from build123d import *

# Parameters (mm, degrees)
SKETCH_1_R      = 1
EXTRUDE_1_DEPTH = 1.5
SKETCH_2_W      = 30
SKETCH_2_H      = 14
EXTRUDE_2_DEPTH = 7.5
SKETCH_3_W      = 8
SKETCH_3_H      = 12
EXTRUDE_3_DEPTH = 5.5


with BuildPart() as part:
    # Эскиз1 → Бобышка-Вытянуть1 (new body)
    with BuildSketch(Plane(origin=(0, 0, 0), x_dir=(1, 0, 0), z_dir=(0, 1, 0))):
        with BuildLine():
            Line((-20, 10), (-12, 10))
            ThreePointArc((-12, 10), (-10, 8), (-8, 10))
            Line((-8, 10), (8, 10))
            ThreePointArc((8, 10), (10, 12), (12, 10))
            Line((12, 10), (20, 10))
            Line((20, 10), (20, 2))
            ThreePointArc((20, 2), (18, 0), (20, -2))
            Line((20, -2), (20, -10))
            Line((20, -10), (12, -10))
            ThreePointArc((12, -10), (10, -12), (8, -10))
            Line((8, -10), (-8, -10))
            ThreePointArc((-8, -10), (-10, -8), (-12, -10))
            Line((-12, -10), (-20, -10))
            Line((-20, -10), (-20, -2))
            ThreePointArc((-20, -2), (-22, 0), (-20, 2))
            Line((-20, 2), (-20, 10))
        make_face()
        with Locations((-20, 0)):
            Circle(SKETCH_1_R, mode=Mode.SUBTRACT)
        with Locations((10, 10)):
            Circle(SKETCH_1_R, mode=Mode.SUBTRACT)
        with Locations((10, -10)):
            Circle(SKETCH_1_R, mode=Mode.SUBTRACT)
    extrude(amount=EXTRUDE_1_DEPTH)

    # Эскиз2 → Бобышка-Вытянуть2 (add)
    with BuildSketch(Plane(origin=(0, 1.5, 0), x_dir=(1, 0, 0), z_dir=(0, 1, 0))):
        with Locations((3, 0)):
            Rectangle(SKETCH_2_W, SKETCH_2_H)
    extrude(amount=EXTRUDE_2_DEPTH)

    # Эскиз3 → Бобышка-Вытянуть3 (add)
    with BuildSketch(Plane.XZ):
        with Locations((16, 0)):
            Rectangle(SKETCH_3_W, SKETCH_3_H)
    extrude(amount=EXTRUDE_3_DEPTH)


solid = part.part
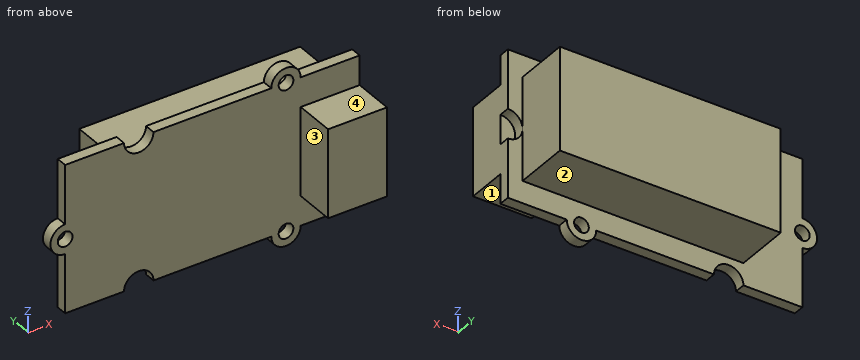
Part model, mm, in its own coordinate system. Face numbers are marked on the shaded views. A direction names the side the tool comes from. Coordinates: 2 decimals unless noted, no trailing zeros. Write each loop counter-clockwise with the first axis right and the second up, starting at its lowest first coordinate (ties: lowest second). Pieces come first, ordered by that corner, then holes. Notation, with made-up numbers: M -9,11.25 L 3,11.25 A9 ccw 3,22.25 Z; hole C 26.5,45 d9. An arc over 180 degrees is marked long. Return JSON: item names as keys, results as strings.
1. Saw through at C-C, the plane x = -5. Write the cut outline in (y, z).
Determined:
{"outline": "M 0,-10 L 1.5,-10 L 1.5,-7 L 9,-7 L 9,7 L 1.5,7 L 1.5,10 L 0,10 Z"}
2. Probe L1, parallel to Z at x = 10, y = 1.15; L2, parallel to X at y = 0.9, z = 0; L3, parallel to Y at x = -2.5, z = 8. List the from-to ranges inside material, lowest first.
Determined:
{"L1": "-12 to -11, -9 to 9, 11 to 12", "L2": "-22 to -21, -19 to 18", "L3": "0 to 1.5"}
3. Saw through at B-B, the plane z = 0.5. Write the cut outline in (x, y), then the cut area to 3 significant figures.
Determined:
{"outline": "M -21.94,0 L -20.87,0 L -20.87,1.5 L -21.94,1.5 Z; M -19.13,0 L 12,0 L 12,-5.5 L 20,-5.5 L 20,0 L 18.06,0 L 18.06,1.5 L 18,1.5 L 18,9 L -12,9 L -12,1.5 L -19.13,1.5 Z", "area": "326 mm²"}
4. Saw through at D-D, the plane y = -3.75. Write the cut outline in (x, z), then the cut area to 3 significant figures.
Determined:
{"outline": "M 12,-6 L 20,-6 L 20,6 L 12,6 Z", "area": "96.0 mm²"}
5. Flat gauge pins, fed straight in: pin 1 Ø3 at (x, y) = (-6, 4.5) entering from +Z; pin 2 Ø1.2 at (x, z) = (10, 10) entering from +Y; pin 3 Ø0.8 at (x, y) = (-2, 0.5) entering from -Z; pin 4 Ø6 at (x, y) = (17, -3.5) entering from -Z. Where does each tip first touch, or does it go through?
Determined:
{"pin 1": "z = 7", "pin 2": "through", "pin 3": "z = -10", "pin 4": "z = -6"}
6. Saw through at A-A, the plane x = 10. Write the cut outline in (y, z).
Determined:
{"outline": "M 0,-12 L 1.5,-12 L 1.5,-11 L 0,-11 Z; M 0,-9 L 1.5,-9 L 1.5,-7 L 9,-7 L 9,7 L 1.5,7 L 1.5,9 L 0,9 Z; M 0,11 L 1.5,11 L 1.5,12 L 0,12 Z"}
7. 3-axis set-ups, long thin cutter, end or side, ignore diameter. For the marked faces 1, 2, 3 and 4: which of +Z, -Z, +X, -X, +Y, -Y reach the whole face in a straight line?
Determined:
{"face 1": "-Z, +X, -X, -Y", "face 2": "-Z, +X, -X, +Y", "face 3": "+Z, -Z, -X, -Y", "face 4": "+Z, +X, -X, -Y"}
